from build123d import *

# Parameters (mm, degrees)
SKETCH3_R          = 1.35
CUT_EXTRUDE2_DEPTH = 34.068111528
CUT_EXTRUDE4_START = -2.5
SKETCH4_R          = 2.25
CUT_EXTRUDE4_DEPTH = 40.058172821
CHAMFER1_SIZE      = 0.1
CIRPATTERN3_COUNT  = 4
CIRPATTERN2_COUNT  = 8


with BuildPart() as part:
    # Sketch7 → Revolve1 (revolve)
    with BuildSketch(Plane(origin=(0, 0, 0), x_dir=(1, 0, 0), z_dir=(0, 1, 0))):
        Polygon((16, 9), (16, 5), (14.5, 5), (14.5, -5), (16, -5), (16, -9), (22.5, -9), (22.5, 9), align=None)
    revolve(axis=Axis((0, 0, 9.9), (0, 0, -1)))

    # Sketch3 → Cut-Extrude2 (cut, symmetric)
    with BuildSketch(Plane.XY):
        with Locations((0, 19.25)):
            Circle(SKETCH3_R)
    cut_extrude2 = extrude(amount=CUT_EXTRUDE2_DEPTH, both=True, mode=Mode.SUBTRACT)

    # Sketch4 → Cut-Extrude4 (cut)
    with BuildSketch(Plane(origin=(0, 0, -9), x_dir=(-1, 0, 0), z_dir=(0, 0, -1)).offset(CUT_EXTRUDE4_START)):
        with Locations(Location((0, 19.25, 0), (0, 0, 180))):
            Circle(SKETCH4_R)
    cut_extrude4 = extrude(amount=CUT_EXTRUDE4_DEPTH, mode=Mode.SUBTRACT)

    # Chamfer1
    chamfer1_edges = [part.edges().sort_by_distance(p)[0] for p in [
        (-1.35, 19.25, -6.5),
    ]]
    chamfer(chamfer1_edges, length=CHAMFER1_SIZE)

    # CirPattern3: Cut-Extrude4 ×4 about axis
    cirpattern3_axis = Axis((0, 0, 0), (0, 0, 1))
    for i in range(1, CIRPATTERN3_COUNT):
        add(cut_extrude4.rotate(cirpattern3_axis, i * 360 / CIRPATTERN3_COUNT), mode=Mode.SUBTRACT)

    # CirPattern2: Cut-Extrude2 ×8 about axis
    cirpattern2_axis = Axis((0, 0, 0), (0, 0, 1))
    for i in range(1, CIRPATTERN2_COUNT):
        add(cut_extrude2.rotate(cirpattern2_axis, i * 360 / CIRPATTERN2_COUNT), mode=Mode.SUBTRACT)


solid = part.part
Input: part model. Units: mm. Frame: model coordinates. A direction names the side the tool comes from. Round coordinates to 2 decimals unless told otherwise and drop trailing zeros. Order: outer loops, then holes, each group sorted by start corner. A loop starts at its lowest first (then second) coordinate and runs counter-clockwise, first axis right, second up. Notation, with made-up numbers: (40.5, 61.25) - (60.5, 61.25) arc R27 ccw to (60.5, 94.25) - close; hole circle Ø10 at (5, 49). An arc over 180 degrees is marked (long way). Use a Markdown table: item, result.
1. Mould query, pull axis Y, two halves, no side actions, for faces 4 (the face through (-3.47, 15.62, 7.03)), 5 (the face through (6.691, 12.864, 0.07)), 6 (the face through (10.382, 19.961, -0.126)), 7 (the face through (7, -15, -9)). Classes: +Y half, -Y half, draft (parallel to the pull), parting line (faces both ways), or undercut.
Evaluation:
| item | result |
|---|---|
| face 4 | undercut |
| face 5 | undercut |
| face 6 | parting line |
| face 7 | draft |
2. Section B-B on y = 19.25. Return the cut outline in (x, z), then the cut area to 3 significant figures.
Evaluation:
| item | result |
|---|---|
| outline | (-11.65, -9) - (-2.25, -9) - (-2.25, -6.5) - (-1.45, -6.5) - (-1.35, -6.4) - (-1.35, 9) - (-11.65, 9) - close; (1.35, -6.4) - (1.45, -6.5) - (2.25, -6.5) - (2.25, -9) - (11.65, -9) - (11.65, 9) - (1.35, 9) - close |
| area | 366 mm^2 |
3. Section D-D on x = -19.25. Return the cut outline in (y, z), then the cut area to 3 significant figures.
Evaluation:
| item | result |
|---|---|
| outline | (-11.65, -9) - (-2.25, -9) - (-2.25, -6.5) - (-1.35, -6.5) - (-1.35, 9) - (-11.65, 9) - close; (1.35, -6.5) - (2.25, -6.5) - (2.25, -9) - (11.65, -9) - (11.65, 9) - (1.35, 9) - close |
| area | 366 mm^2 |
4. Section C-C on z = 1.5. State how many separate pieces and enclosed holes the cut face has, then the cut area to 3 significant figures.
Evaluation:
| item | result |
|---|---|
| separate pieces | 1 |
| enclosed holes | 9 |
| area | 884 mm^2 |
5. Material intervals for probe 1 along Y at (x, z) = (0, -7.4); probe 2 along Y at (x, z) = (0, 5.25), sorted ascending.
Evaluation:
| item | result |
|---|---|
| probe 1 | -22.5 to -21.5, -17 to -16, 16 to 17, 21.5 to 22.5 |
| probe 2 | -22.5 to -20.6, -17.9 to -16, 16 to 17.9, 20.6 to 22.5 |
6. First-contact query: pin 1 (1 mm diameter, centred on x = 7.5, z = -2, fed in from +Y); pin 2 (3.5 mm diameter, centred on x = -19.25, y = 0, fed in from +Z); pin 3 (2 mm diameter, centred on x = 18.5, y = -0.5, fed in from -Z); pin 4 (2.5 mm diameter, centred on x = 0, y = -19.25, fed in from +Z). Flat tips, straight axial feed; report the tip coordinate or a pass-through.
Evaluation:
| item | result |
|---|---|
| pin 1 | y = 21.38 |
| pin 2 | z = 9 |
| pin 3 | z = -6.5 |
| pin 4 | through |
7. Access query for faces 1 (the face through (0, 21, -6.5)), 2 (the face through (3.6, -14.3, 5)), 3 (the face through (-18.05, 0.62, 1.36)). Directions: +Z, -Z, +X, -X, +Y, -Y. A direction counts if a zero-diameter tool reaches every point of the face in a straight line with its end or side. Return the directions, or none.
Evaluation:
| item | result |
|---|---|
| face 1 | -Z |
| face 2 | +Z |
| face 3 | +Z, -Z |
8. Section A-A on x = 5. Return the cut outline in (y, z), then the cut area to 3 significant figures.
Evaluation:
| item | result |
|---|---|
| outline | (-21.94, -9) - (-15.2, -9) - (-15.2, -5) - (-13.61, -5) - (-13.61, 5) - (-15.2, 5) - (-15.2, 9) - (-21.94, 9) - close; (13.61, -5) - (15.2, -5) - (15.2, -9) - (21.94, -9) - (21.94, 9) - (15.2, 9) - (15.2, 5) - (13.61, 5) - close |
| area | 274 mm^2 |
